CAD build for the part. Positions are in the model's coordinates, mm. Face numbers are marked on the shaded views. Coordinates: 2 decimals unless noted, no trailing zeros. Loops run counter-clockwise (first coordinate to the right, second up) from the corner with the lowest first, then second, coordinate; pieces in that order, holes last. Notation, with made-up numbers: (53.5, -19) -> (74.5, -19) arc R12 ccw to (74.5, 0) -> close; hole circle Ø1 at (89.25, 10). An arc over 180 degrees is marked (long way). Write each question's results on one line, items separated by ' | '.
from build123d import *

# Parameters (mm, degrees)
SKETCH_R     = 51.661794
SKETCH_R_2   = 7.362217
SKETCH_R_3   = 9.837508
PAD_DEPTH    = 10
POCKET_DEPTH = 3
PAD001_DEPTH = 10


with BuildPart() as part:
    # Sketch → Pad (new body)
    with BuildSketch(Plane.XY):
        Circle(SKETCH_R)
        with Locations((-22.600981, 24.427324)):
            Circle(SKETCH_R_2, mode=Mode.SUBTRACT)
        with Locations((15.600001, 29.601961)):
            Circle(SKETCH_R_3, mode=Mode.SUBTRACT)
    extrude(amount=PAD_DEPTH)

    # Sketch001 → Pocket (cut)
    with BuildSketch(Plane.XY.offset(10)):
        Polygon((-10.425369, -26.558058), (8.446838, -21.840006), (18.491709, -9.664394), (13.012688, -31.732695), align=None)
    extrude(amount=-POCKET_DEPTH, mode=Mode.SUBTRACT)

    # Sketch002 → Pad001 (new body)
    with BuildSketch(Plane.XY.offset(10)):
        Polygon((-6.599153, -7.156828), (2.509538, 10.131093), (10.50287, -4.740234), align=None)
    extrude(amount=PAD001_DEPTH)


solid = part.part
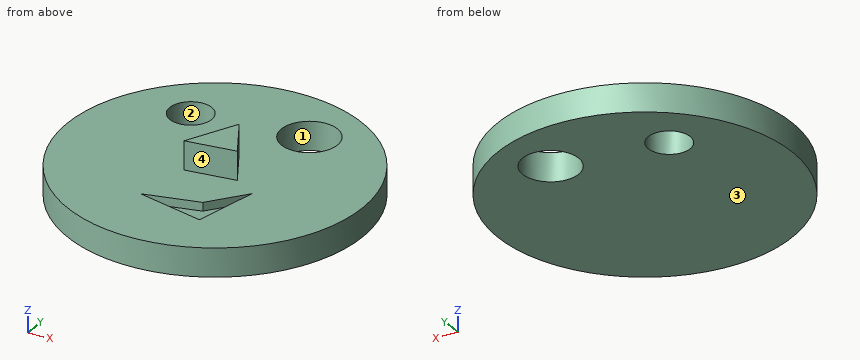
1) Pin check, flat tips, straight feed: pin 1 (17.5 mm diameter, centred on x = 6.5, y = -26, fed in from +Z); pin 2 (2 mm diameter, centred on x = 6, z = 7.5, fed in from +Y); pin 3 (1.5 mm diameter, centred on x = 32.5, z = 7, fed in from -Y). Stop position of each tip, or through.
Outcome:
pin 1: stops at z = 10 | pin 2: stops at y = 51.42 | pin 3: stops at y = -40.75
2) Slice it at B-B (z = 8.5). Write the cut outline in (x, y), then the cut area to 3 significant figures.
Outcome:
outline: circle Ø103.32 at (0, 0); hole circle Ø14.72 at (-22.6, 24.43); hole (-10.43, -26.56) -> (13.01, -31.73) -> (18.49, -9.66) -> (8.45, -21.84) -> close; hole circle Ø19.68 at (15.6, 29.6) | area: 7,730 mm^2
3) Two-plate mould, pull along X, no slides. Class the marked faces 1, 2, 3 and 4: pulls with the +X half, pulls with the -X half, needs draft (parallel to the pull), parting line crosses it, or undercut.
Outcome:
face 1: undercut | face 2: undercut | face 3: needs draft | face 4: pulls with the +X half
4) Drill centre lines: L1, parallel to X at y = 27, z = 5.5; L2, parallel to Y at x = 8, z = 8.75; L3, parallel to Z at x = -42.5, y = 15. Where is each one in solid material? Low to high. Write a range as from..to.
Outcome:
L1: x = -44.04..-29.5, -15.7..6.11, 25.09..44.04 | L2: y = -51.04..-30.63, -21.95..23.36, 35.85..51.04 | L3: z = 0..10
5) Slice it at A-A (x = 7). Write the cut outline in (y, z), then the cut area to 3 significant figures.
Outcome:
outline: (-51.19, 0) -> (24.83, 0) -> (24.83, 10) -> (1.78, 10) -> (1.78, 20) -> (-5.24, 20) -> (-5.24, 10) -> (-22.2, 10) -> (-22.2, 7) -> (-30.41, 7) -> (-30.41, 10) -> (-51.19, 10) -> close; (34.38, 0) -> (51.19, 0) -> (51.19, 10) -> (34.38, 10) -> close | area: 974 mm^2
6) Slice it at C-C (y = -14). Write the cut outline in (x, z), then the cut area to 3 significant figures.
Outcome:
outline: (-49.73, 0) -> (49.73, 0) -> (49.73, 10) -> (17.42, 10) -> (17.42, 7) -> (14.91, 7) -> (14.91, 10) -> (-49.73, 10) -> close | area: 987 mm^2
7) Slice it at D-D (z = 16.5). Write the cut outline in (x, y).
Outcome:
outline: (-6.6, -7.16) -> (10.5, -4.74) -> (2.51, 10.13) -> close
